from build123d import *

# Parameters (mm, degrees)
SKETCH1_R           = 20
BOSS_EXTRUDE1_DEPTH = 71
SKETCH2_R           = 8
BOSS_EXTRUDE2_DEPTH = 1.4
SKETCH3_R           = 4
BOSS_EXTRUDE3_DEPTH = 2.15
SKETCH4_R           = 3
BOSS_EXTRUDE4_DEPTH = 20.3
SKETCH5_R           = 1
SKETCH5_R_2         = 0.8
CUT_EXTRUDE1_DEPTH  = 3
CUT_EXTRUDE2_DEPTH  = 1
BOSS_EXTRUDE5_DEPTH = 8
SKETCH8_R           = 2.75
CUT_EXTRUDE3_DEPTH  = 0.5
CUT_EXTRUDE4_REACH  = 40.687
SKETCH9_R           = 1
CUT_EXTRUDE5_START  = -31.9
SKETCH9_2_R         = 1
CUT_EXTRUDE5_DEPTH  = 0.5
SKETCH10_R          = 1.5
SKETCH10_R_2        = 1.75
CUT_EXTRUDE6_DEPTH  = 5


with BuildPart() as part:
    # Sketch1 → Boss-Extrude1 (new body)
    with BuildSketch(Plane.XY):
        Circle(SKETCH1_R)
    extrude(amount=BOSS_EXTRUDE1_DEPTH)

    # Sketch2 → Boss-Extrude2 (add)
    with BuildSketch(Plane.XY.offset(71)):
        Circle(SKETCH2_R)
    extrude(amount=BOSS_EXTRUDE2_DEPTH)

    # Sketch3 → Boss-Extrude3 (add)
    with BuildSketch(Plane.XY.offset(72.4)):
        Circle(SKETCH3_R)
    extrude(amount=BOSS_EXTRUDE3_DEPTH)

    # Sketch4 → Boss-Extrude4 (add)
    with BuildSketch(Plane.XY.offset(74.55)):
        Circle(SKETCH4_R)
    extrude(amount=BOSS_EXTRUDE4_DEPTH)

    # Sketch5 → Cut-Extrude1 (cut)
    with BuildSketch(Plane.XY.offset(71)):
        with Locations((12.218624281, 9.041306359)):
            Circle(SKETCH5_R)
        with Locations((-12.218624281, -9.041306359)):
            Circle(SKETCH5_R)
        with Locations((-1.720688849, 15.102292206)):
            Circle(SKETCH5_R)
        with Locations((1.720688849, -15.102292206)):
            Circle(SKETCH5_R)
        with Locations((10.20898213, 7.554249392)):
            Circle(SKETCH5_R_2)
        with Locations((-10.20898213, -7.554249392)):
            Circle(SKETCH5_R_2)
    extrude(amount=-CUT_EXTRUDE1_DEPTH, mode=Mode.SUBTRACT)

    # Sketch6 → Cut-Extrude2 (cut)
    with BuildSketch(Plane.XY.offset(71)):
        Polygon((-19.987250443, 1.571566014), (-12.76743464, 0.492557313), (-12.353568289, 3.26180173), (-19.573384092, 4.340810431), align=None)
        Polygon((19.573384092, -4.340810431), (12.353568289, -3.26180173), (12.76743464, -0.492557313), (19.987250443, -1.571566014), align=None)
    extrude(amount=-CUT_EXTRUDE2_DEPTH, mode=Mode.SUBTRACT)

    # Sketch7 → Boss-Extrude5 (add)
    with BuildSketch(Plane.XY.offset(70)):
        Polygon((-15.981736196, 0.972937899), (-15.567869845, 3.742182316), (-15.073361913, 3.668277611), (-15.487228265, 0.899033193), align=None)
        Polygon((15.567869845, -3.742182316), (15.981736196, -0.972937899), (15.487228265, -0.899033193), (15.073361913, -3.668277611), align=None)
    extrude(amount=BOSS_EXTRUDE5_DEPTH)

    # Sketch8 → Cut-Extrude3 (cut)
    with BuildSketch(Plane.XY.offset(71)):
        with Locations((8.199604269, 11.285787072)):
            Circle(SKETCH8_R)
        with Locations((-8.199604269, -11.285787072)):
            Circle(SKETCH8_R)
    extrude(amount=-CUT_EXTRUDE3_DEPTH, mode=Mode.SUBTRACT)

    # Sketch9 → Cut-Extrude4 (cut, up to next)
    with BuildSketch(Plane(origin=(15.774803021, -2.357560108, 0), x_dir=(0, 0, -1), z_dir=(0.989015863, -0.147809411, 0)), mode=Mode.PRIVATE) as cut_extrude4_sk1:
        with Locations((-75, 0)):
            Circle(SKETCH9_R)
    cut_extrude4_tool1 = extrude(cut_extrude4_sk1.sketch, amount=-CUT_EXTRUDE4_REACH, mode=Mode.PRIVATE) & part.part
    add(cut_extrude4_tool1.solids().sort_by_distance((15.774803, -2.35756, 75))[0], mode=Mode.SUBTRACT)

    # Sketch9_2 → Cut-Extrude5 (cut)
    with BuildSketch(Plane(origin=(15.774803021, -2.357560108, 0), x_dir=(0, 0, -1), z_dir=(0.989015863, -0.147809411, 0)).offset(CUT_EXTRUDE5_START)):
        with Locations((-75, 0)):
            Circle(SKETCH9_2_R)
    extrude(amount=CUT_EXTRUDE5_DEPTH, mode=Mode.SUBTRACT)

    # Sketch10 → Cut-Extrude6 (cut)
    with BuildSketch(Plane(origin=(0, 0, 0), x_dir=(-1, 0, 0), z_dir=(0, 0, -1))):
        with Locations((0, 11)):
            Circle(SKETCH10_R)
        with Locations((9.526279442, 5.5)):
            Circle(SKETCH10_R)
        with Locations((9.526279442, -5.5)):
            Circle(SKETCH10_R)
        with Locations((0, -11)):
            Circle(SKETCH10_R)
        with Locations((-9.526279442, -5.5)):
            Circle(SKETCH10_R)
        with Locations((-9.526279442, 5.5)):
            Circle(SKETCH10_R)
        with Locations((0, 16)):
            Circle(SKETCH10_R_2)
    extrude(amount=-CUT_EXTRUDE6_DEPTH, mode=Mode.SUBTRACT)


solid = part.part
For this review, take the finished solid that the model builds, in its own axes (mm). A direction names the side the tool comes from. Round coordinates to 2 decimals unless told otherwise and drop trailing zeros. Loops run counter-clockwise (first coordinate to the right, second up) from the corner with the lowest first, then second, coordinate; pieces in that order, holes last. Notation, with made-up numbers: (74.25, 69) - (83.25, 69) arc R15 ccw to (83.25, 73) - close; hole circle Ø4 at (30, -14). An arc over 180 degrees is marked (long way). Use one line per item in the form item = value.
Item 1: Tool access review of faces 1 (the flat face through (-15.185, 2.918, 73.944)), 2 (the cylindrical face through (0.228, 17.735, 2.465)), 3 (the cylindrical face through (15.5, -2.3, 76)): name each direction out of +Z, -Z, +X, -X, +Y, -Y from which nothing blocks a thin tool from reaching the whole face with its end or side.
Answers:
face_1 = +Z
face_2 = -Z
face_3 = none
Item 2: Clearance check with flat-ended pins moving along their axes: P1, Ø1.7, axis at x = 17.5, y = -3, coming from the +Z side; P2, Ø2.5, axis at x = 9.53, y = -5.5, coming from the -Z side; P3, Ø3.5, axis at x = -9.53, y = -5.5, coming from the +Z side. State where each tip first meets the part, or that it passes through.
Answers:
P1 = 70
P2 = 5
P3 = 71
Item 3: Consider section B-B on z = 20. Write out the cut boundary in (x, y), then the cut area to 3 significant figures.
Answers:
outline = circle Ø40 at (0, 0)
area = 1,260 mm^2
Item 4: Consider section C-C on z = 81.5. Write out the cut boundary in (x, y), then the cut area to 3 significant figures.
Answers:
outline = circle Ø6 at (0, 0)
area = 28.3 mm^2
Item 5: Consider section A-A on y = 5.5. Write out the cut boundary in (x, z).
Answers:
outline = (-19.23, 0) - (-11.03, 0) - (-11.03, 5) - (-8.03, 5) - (-8.03, 0) - (8.03, 0) - (8.03, 5) - (11.03, 5) - (11.03, 0) - (19.23, 0) - (19.23, 71) - (5.81, 71) - (5.81, 72.4) - (-5.81, 72.4) - (-5.81, 71) - (-19.23, 71) - close
Item 6: For line 1 (Z direction, x = -9.5, y = 7.5); line 2 (Z direction, x = 7, y = 2.5); line 3 (X direction, y = 2.5, z = 75), list the stretches that pass through material, from the lowest coordinate up.
Answers:
line_1 = 0 to 71
line_2 = 0 to 72.4
line_3 = -1.66 to 1.66
